from build123d import *

# Parameters (mm, degrees)
IZIM1_R                     = 3
IZIM1_R_2                   = 1.5
Y_KSEKLIK_EKSTR_ZYON1_DEPTH = 2


with BuildPart() as part:
    # Çizim1 → Yükseklik-Ekstrüzyon1 (new body)
    with BuildSketch(Plane(origin=(0, 0, 0), x_dir=(1, 0, 0), z_dir=(0, 1, 0))):
        with BuildLine():
            Line((-80, 55), (-73.768114575, 55))
            ThreePointArc((-73.768114575, 55), (-73, 49.1), (-72.231885425, 55))
            Line((-72.231885425, 55), (77, 55))
            ThreePointArc((77, 55), (74.878679656, 49.878679656), (80, 52))
            Line((80, 52), (80, -50.841687605))
            ThreePointArc((80, -50.841687605), (75.378679656, -50.378679656), (75.841687605, -55))
            Line((75.841687605, -55), (-77, -55))
            ThreePointArc((-77, -55), (-77.878679656, -52.878679656), (-80, -52))
            Line((-80, -52), (-80, 55))
        make_face()
        with Locations(Location((7, -35.5, 0), (0, 0, 270))):
            Circle(IZIM1_R, mode=Mode.SUBTRACT)
        with Locations(Location((3, 13, 0), (0, 0, 270))):
            Circle(IZIM1_R, mode=Mode.SUBTRACT)
        with Locations(Location((-33, -45, 0), (0, 0, 270))):
            Circle(IZIM1_R_2, mode=Mode.SUBTRACT)
        with Locations(Location((-7.88, -45, 0), (0, 0, 270))):
            Circle(IZIM1_R_2, mode=Mode.SUBTRACT)
        with Locations(Location((7, -45, 0), (0, 0, 270))):
            Circle(IZIM1_R_2, mode=Mode.SUBTRACT)
        with Locations(Location((32.12, -45, 0), (0, 0, 270))):
            Circle(IZIM1_R_2, mode=Mode.SUBTRACT)
        with Locations(Location((-55.5, -53, 0), (0, 0, 270))):
            Circle(IZIM1_R_2, mode=Mode.SUBTRACT)
        with Locations(Location((-43.3, -53, 0), (0, 0, 270))):
            Circle(IZIM1_R_2, mode=Mode.SUBTRACT)
    extrude(amount=Y_KSEKLIK_EKSTR_ZYON1_DEPTH)


solid = part.part
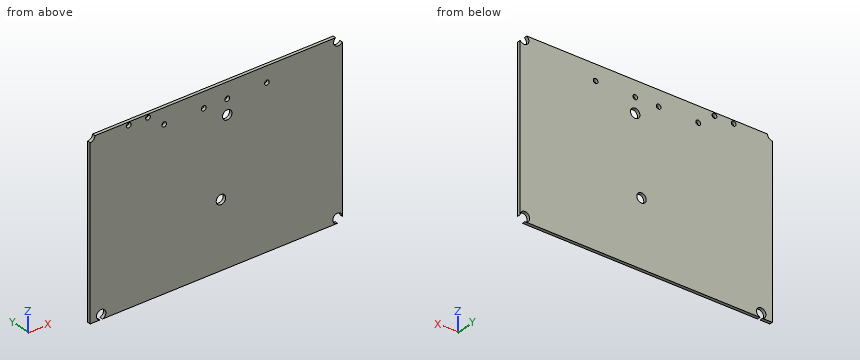
CAD build for the part. Positions are in the model's coordinates, mm. Round coordinates to 2 decimals unless told otherwise and drop trailing zeros. Loops run counter-clockwise (first coordinate to the right, second up) from the corner with the lowest first, then second, coordinate; pieces in that order, holes last. Notation, with made-up numbers: M 22,61 L 71,61 A21 cw 71,83 Z; hole C 63,36 d5. An arc over 180 degrees is marked long. One line per question, with ' | ' between items. Start each with the question number.
Item 1: Pin check, flat tip, straight feed: pin 1 Ø7 at (x, z) = (7, 35.5) entering from -Y. Stop position of the tip, or through.
Item 2: Cut at A-A, the plane z = 35.5. Write the cut outline in (x, y), plus the area to 3 significant figures.
Item 3: Wall check: line 1 (X direction, y = 1.45, z = 35.5); line 2 (X direction, y = 1, z = -49.5); line 3 (X direction, y = 0.6, z = 45). Give the ranges that are in metal, low to high.
Responses:
1) pin 1: stops at y = 0
2) outline: M -80,0 L 4,0 L 4,2 L -80,2 Z; M 10,0 L 80,0 L 80,2 L 10,2 Z | area: 308 mm²
3) line 1: x = -80 to 4, 10 to 80 | line 2: x = -80 to -74.5, -71.5 to 75.34, 78.66 to 80 | line 3: x = -80 to -34.5, -31.5 to -9.38, -6.38 to 5.5, 8.5 to 30.62, 33.62 to 80
